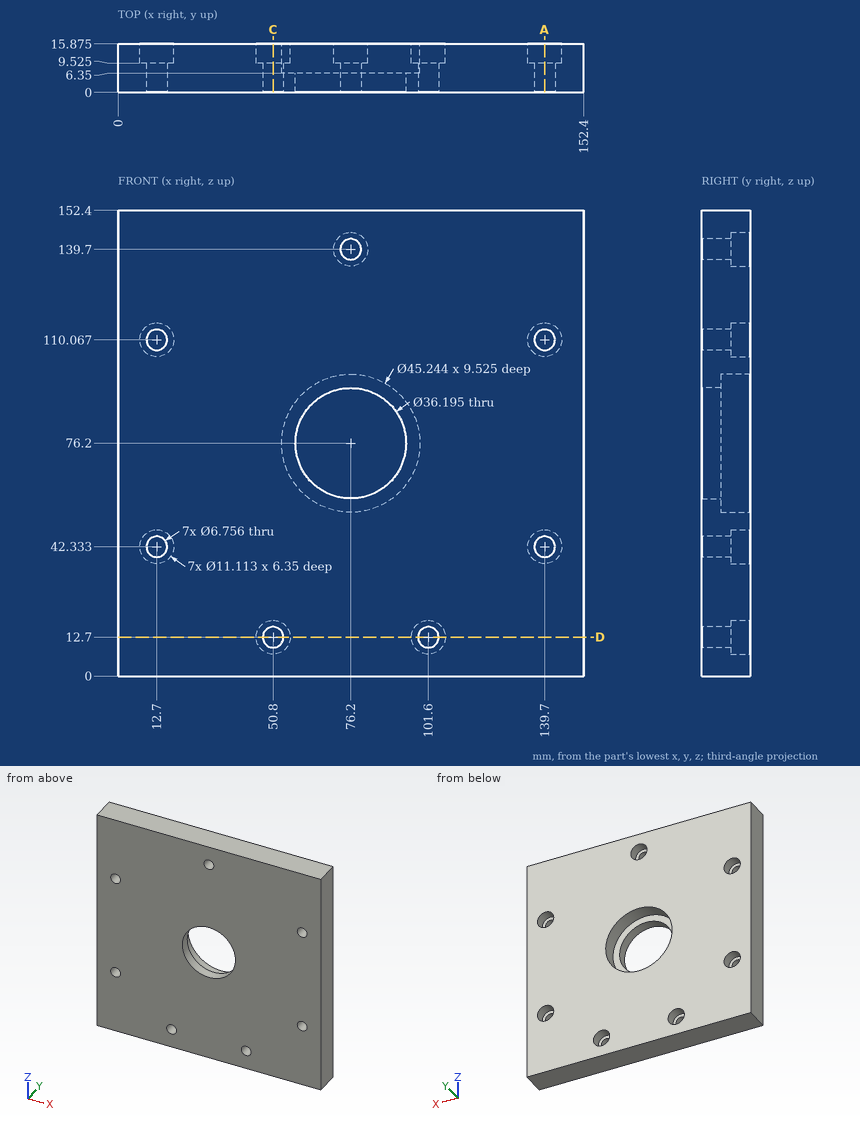
For this review, use the dimensioned drawing (mm, ordinates from the lowest corner) and the shaded views. Round coordinates to 2 decimals unless told otherwise and drop trailing zeros. Order: outer loops, then holes, each group sorted by start corner. A loop starts at its lowest first (then second) coordinate and runs counter-clockwise, first axis right, second up.
1) Consider section A-A (x = 139.7). State the section outline as (y, z) points (1 decimal).
The answers:
outline: (0, 0) - (15.9, 0) - (15.9, 36.8) - (9.5, 36.8) - (9.5, 39) - (0, 39) - close; (0, 45.7) - (9.5, 45.7) - (9.5, 47.9) - (15.9, 47.9) - (15.9, 104.5) - (9.5, 104.5) - (9.5, 106.7) - (0, 106.7) - close; (0, 113.4) - (9.5, 113.4) - (9.5, 115.6) - (15.9, 115.6) - (15.9, 152.4) - (0, 152.4) - close
2) Consider section C-C (x = 50.8). State the section outline as (y, z) points (1 decimal), plus the area to 3 significant figures.
The answers:
outline: (0, 0) - (15.9, 0) - (15.9, 7.1) - (9.5, 7.1) - (9.5, 9.3) - (0, 9.3) - close; (0, 16.1) - (9.5, 16.1) - (9.5, 18.3) - (15.9, 18.3) - (15.9, 152.4) - (0, 152.4) - close
area: 2,280 mm2
3) Clearance check with flat-ended pins moving along their axes: pin 1 Ø3.5 at (x, z) = (140.5, 40.5) entering from +Y (1 decimal); pin 2 Ø4 at (x, z) = (12.7, 42.33) entering from +Y. State where each tip first meets the part, or that it passes through.
The answers:
pin 1: stops at y = 9.5
pin 2: passes through
4) For L1, parallel to X at y = 3.5, z = 12.7; L2, parallel to Z at x = 139.7, y = 5 (1 decimal); L3, parallel to Z at x = 76.5, y = 8.25 (1 decimal), list the stretches that pass through material, from the lowest coordinate up.
The answers:
L1: x = 0 to 47.42, 54.18 to 98.22, 104.98 to 152.4
L2: z = 0 to 39, 45.7 to 106.7, 113.4 to 152.4
L3: z = 0 to 53.6, 98.8 to 136.3, 143.1 to 152.4
5) Consider section D-D (z = 12.7). State the section outline as (x, y) points (1 decimal), plus the area to 3 significant figures.
The answers:
outline: (0, 0) - (47.4, 0) - (47.4, 9.5) - (45.2, 9.5) - (45.2, 15.9) - (0, 15.9) - close; (54.2, 0) - (98.2, 0) - (98.2, 9.5) - (96, 9.5) - (96, 15.9) - (56.4, 15.9) - (56.4, 9.5) - (54.2, 9.5) - close; (105, 0) - (152.4, 0) - (152.4, 15.9) - (107.2, 15.9) - (107.2, 9.5) - (105, 9.5) - close
area: 2,150 mm2
